Source: CAD feature listing. Evaluate the final solid. Frame: model axes, mm. Face numbers are marked on the shaded views. A direction names the side the tool comes from. Round coordinates to 2 decimals unless told otherwise and drop trailing zeros. Loops run counter-clockwise (first coordinate to the right, second up) from the corner with the lowest first, then second, coordinate; pieces in that order, holes last. Notation, with made-up numbers: (-8, 73.25) - (34, 73.25) arc R34 cw to (34, 108.25) - close; hole circle Ø3 at (83.5, 56.25). An arc over 180 degrees is marked (long way). One line per question, with ' | ' between items.
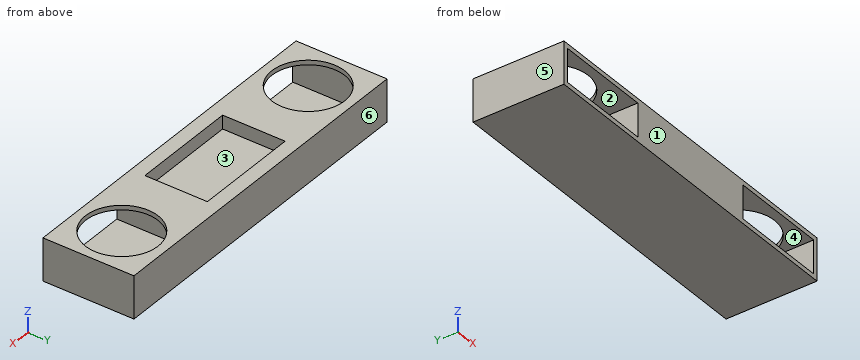
from build123d import *

# Parameters (mm, degrees)
F0_W     = 1447.8
F0_H     = 381
F1_DEPTH = 177.8
F4_T     = -19.05
F2_R     = 152.4
F5_DEPTH = 25.4
F3_W     = 603.25
F3_H     = 177.8
F6_DEPTH = 381
F2_W     = 444.5
F2_H     = 261.9375
F7_DEPTH = 57.15


with BuildPart() as f1:
    # F0 (on Top) → F1 (new body)
    with BuildSketch(Plane.XY):
        Rectangle(F0_W, F0_H)
    extrude(amount=F1_DEPTH)

    # F4
    f4_openings = [f1.faces().sort_by_distance(p)[0] for p in [
        (0, -190.5, 88.9),
    ]]
    offset(amount=F4_T, openings=f4_openings)

    # F2 (on face) → F5 (cut)
    with BuildSketch(Plane.XY.offset(177.8)):
        with Locations((-533.4, 0)):
            Circle(F2_R)
        with Locations((533.4, 0)):
            Circle(F2_R)
    extrude(amount=-F5_DEPTH, mode=Mode.SUBTRACT)

    # F3 (on face) → F6 (join)
    with BuildSketch(Plane.XZ.offset(190.5)):
        with Locations((0, 88.9)):
            Rectangle(F3_W, F3_H)
    extrude(amount=-F6_DEPTH)

    # F2 (on face) → F7 (cut)
    with BuildSketch(Plane.XY.offset(177.8)):
        Rectangle(F2_W, F2_H)
    extrude(amount=-F7_DEPTH, mode=Mode.SUBTRACT)


solid = f1.part
1. Section query B-B, the plane z = 144. Return loops of the section in (x, y) (3 decimals), plus the area to 3 significant figures.
Worked out:
outline: (-723.9, -190.5) - (-704.85, -190.5) - (-704.85, 171.45) - (-301.625, 171.45) - (-301.625, -190.5) - (301.625, -190.5) - (301.625, 171.45) - (704.85, 171.45) - (704.85, -190.5) - (723.9, -190.5) - (723.9, 190.5) - (-723.9, 190.5) - close; hole (-222.25, -130.969) - (222.25, -130.969) - (222.25, 130.969) - (-222.25, 130.969) - close | area: 143,000 mm2
2. Contact query for flat-ended pins moving along their axis: P1, Ø10, axis at x = -248.5, y = 97.5, coming from the -Z side; P2, Ø6, axis at x = -202.5, y = 99.5, coming from the +Z side; P3, Ø10, axis at x = 530.5, y = 59.5, coming from the +Z side; P4, Ø2, axis at x = 432, z = 41.5, coming from the -Y side. Output: stop coordinate, or through.
Worked out:
P1: stops at z = 0 | P2: stops at z = 120.65 | P3: stops at z = 19.05 | P4: stops at y = 171.45
3. Access query for the marked faces 1, 2 and 3. Directions: +Z, -Z, +X, -X, +Y, -Y. A direction counts if a zero-diameter tool reaches every point of the face in a straight line with its end or side. Return the directions, or none.
Worked out:
face 1: +Z, -Z, +X, -X, -Y | face 2: -Y | face 3: +Z
4. Mould query, pull axis X, two halves, no side actions, for the marked faces 4, 5 and 6. Classes: released by +X, released by -X, zero draft, split by the parting line, or undercut.
Worked out:
face 4: undercut | face 5: released by -X | face 6: zero draft
5. Section query C-C, the plane x = 151.5. Return loops of the section in (y, z), plus the area to 3 significant figures.
Worked out:
outline: (-190.5, 0) - (190.5, 0) - (190.5, 177.8) - (130.97, 177.8) - (130.97, 120.65) - (-130.97, 120.65) - (-130.97, 177.8) - (-190.5, 177.8) - close | area: 52,800 mm2
6. Section query A-A, the plane x = -533.4. Return loops of the section in (y, z), plus the area to 3 significant figures.
Worked out:
outline: (-190.5, 0) - (190.5, 0) - (190.5, 177.8) - (152.4, 177.8) - (152.4, 158.75) - (171.45, 158.75) - (171.45, 19.05) - (-190.5, 19.05) - close; (-190.5, 158.75) - (-152.4, 158.75) - (-152.4, 177.8) - (-190.5, 177.8) - close | area: 11,400 mm2
7. Material intervals for probe 1 along X at (y, z) = (141, 135) (3 decimals); probe 2 along X at (y, z) = (119, 123) (3 decimals); probe 3 along Y at (x, z) = (-533.4, 163.5), sorted ascending.
Worked out:
probe 1: x = -723.9 to -704.85, -301.625 to 301.625, 704.85 to 723.9 | probe 2: x = -723.9 to -704.85, -301.625 to -222.25, 222.25 to 301.625, 704.85 to 723.9 | probe 3: y = -190.5 to -152.4, 152.4 to 190.5
8. Section query D-D, the plane y = 0. Return loops of the section in (x, z) (3 decimals), plus the area to 3 significant figures.
Worked out:
outline: (-723.9, 0) - (723.9, 0) - (723.9, 177.8) - (685.8, 177.8) - (685.8, 158.75) - (704.85, 158.75) - (704.85, 19.05) - (301.625, 19.05) - (301.625, 158.75) - (381, 158.75) - (381, 177.8) - (222.25, 177.8) - (222.25, 120.65) - (-222.25, 120.65) - (-222.25, 177.8) - (-381, 177.8) - (-381, 158.75) - (-301.625, 158.75) - (-301.625, 19.05) - (-704.85, 19.05) - (-704.85, 158.75) - (-685.8, 158.75) - (-685.8, 177.8) - (-723.9, 177.8) - close | area: 108,000 mm2
